Source: CAD feature listing. Evaluate the final solid. Frame: model axes, mm. A direction names the side the tool comes from. Coordinates: 2 decimals unless noted, no trailing zeros. Loops run counter-clockwise (first coordinate to the right, second up) from the corner with the lowest first, then second, coordinate; pieces in that order, holes last. Notation, with made-up numbers: M 57.5,86 L 68.5,86 A22 cw 68.5,123 Z; hole C 47.5,56 d11. An arc over 180 degrees is marked long. Write each question's results on one line, items separated by ' | '. Start each with the question number.
from build123d import *

# Parameters (mm, degrees)
F1_DEPTH  = 20
F2_R      = 3
F4_DEPTH  = 10.001
F5_DEPTH  = 6.5
F6_ANGLE  = -90
F7_R      = 2.25
F8_DEPTH  = 5.5
F9_R      = 3.75
F9_R_2    = 2.25
F10_DEPTH = 4


with BuildPart() as f1:
    # F0 (on Top) → F1 (new body)
    with BuildSketch(Plane.XY):
        Polygon((-15.7, 0), (0, 0), (15.7, 0), (15.7, 29.4), (10.2, 29.4), (9.7, 28), (10.2, 27.4), (10.2, 8), (3.1, 8), (2.1, 10), (0, 10), (-2.1, 10), (-3.1, 8), (-10.2, 8), (-10.2, 27.4), (-9.7, 28), (-10.2, 29.4), (-15.7, 29.4), align=None)
    extrude(amount=F1_DEPTH)

    # F2
    f2_edges = [f1.edges().sort_by_distance(p)[0] for p in [
        (12.95, 29.4, 20),
        (-12.95, 29.4, 20),
        (-12.95, 29.4, 0),
        (12.95, 29.4, 0),
    ]]
    fillet(f2_edges, radius=F2_R)

    # F3 (on face) → F4 (cut, through all)
    with BuildSketch(Plane(origin=(0, 10, 0), x_dir=(-1, 0, 0), z_dir=(0, 1, 0))):
        with BuildLine():
            ThreePointArc((5.95, 10), (4.5551315688, 12.0811655388), (2.1, 11.581929202))
            Line((2.1, 11.581929202), (2.1, 8.418070798))
            ThreePointArc((2.1, 8.418070798), (4.5551315688, 7.9188344612), (5.95, 10))
        make_face()
        with BuildLine():
            Line((2.1, 8.418070798), (2.1, 11.581929202))
            ThreePointArc((2.1, 11.581929202), (1.45, 10), (2.1, 8.418070798))
        make_face()
    extrude(amount=-F4_DEPTH, mode=Mode.SUBTRACT)

    # F3 (on face) → F5 (cut)
    with BuildSketch(Plane(origin=(0, 10, 0), x_dir=(-1, 0, 0), z_dir=(0, 1, 0))):
        with BuildLine():
            ThreePointArc((2.1, 6.6084664236), (5.7077973005, 6.8327851352), (7.45, 10))
            ThreePointArc((7.45, 10), (5.7077973005, 13.1672148648), (2.1, 13.3915335764))
            Line((2.1, 13.3915335764), (2.1, 11.581929202))
            ThreePointArc((2.1, 11.581929202), (4.5551315688, 12.0811655388), (5.95, 10))
            ThreePointArc((5.95, 10), (4.5551315688, 7.9188344612), (2.1, 8.418070798))
            Line((2.1, 8.418070798), (2.1, 6.6084664236))
        make_face()
        with BuildLine():
            Line((2.1, 11.581929202), (2.1, 13.3915335764))
            ThreePointArc((2.1, 13.3915335764), (-0.05, 10), (2.1, 6.6084664236))
            Line((2.1, 6.6084664236), (2.1, 8.418070798))
            ThreePointArc((2.1, 8.418070798), (1.45, 10), (2.1, 11.581929202))
        make_face()
    extrude(amount=-F5_DEPTH, mode=Mode.SUBTRACT)


with BuildPart() as f1_1:
    # F6: moved
    add(f1.part.rotate(Axis((0, 0, 0), (-1, 0, 0)), F6_ANGLE))

    # F7 (on face) → F8 (cut, through all)
    with BuildSketch(Plane.YZ.offset(-10.2)):
        with Locations((-10, 18)):
            Circle(F7_R)
    extrude(amount=-F8_DEPTH, mode=Mode.SUBTRACT)

    # F9 (on face) → F10 (cut)
    with BuildSketch(Plane(origin=(-15.7, 0, 0), x_dir=(0, -1, 0), z_dir=(-1, 0, 0))):
        with Locations((10, 18)):
            Circle(F9_R)
        with Locations((10, 18)):
            Circle(F9_R_2, mode=Mode.SUBTRACT)
    extrude(amount=-F10_DEPTH, mode=Mode.SUBTRACT)


solid = f1_1.part
Item 1: Line query: probe 1 along X at (y, z) = (-10, 2.5); probe 2 along X at (y, z) = (-14, 18.5); probe 3 along Z at (x, y) = (-11, -10). Output: solid intervals per line, ascending.
Item 2: Cut plane C-C (z = 5.5). Output: boundary loops of the cut face in (x, y), then the cut area to 3 significant figures.
Item 3: Access query for faces 1 (the cylindrical face through (-13.73, -9.19, 14.34)), 2 (the flat face through (-9.946, -9.866, 28.69)), 3 (the flat face through (-3.6, -7.6, 3.5)), 4 (the flat face through (-8, -10, 8)), 5 (the cylindrical face through (-12.74, -0.9, 28.54)). Directions: +Z, -Z, +X, -X, +Y, -Y. A direction counts if a zero-diameter tool reaches every point of the face in a straight line with its end or side. Return the directions, or none.
Item 4: Cut plane D-D (y = -4.75). Output: boundary loops of the cut face in (x, z).
Item 5: First-contact query: pin 1 Ø2 at (x, y) = (-4.5, -10.5) entering from +Z (3 decimals); pin 2 Ø3.5 at (x, y) = (6, -13.5) entering from +Z; pin 3 Ø1.3 at (x, y) = (1, -8.5) entering from +Z. Flat tips, straight axial feed; report the tip coordinate or a pass-through.
Item 6: Cut plane A-A (z = 12.75). Output: boundary loops of the cut face in (x, y), then the cut area to 3 significant figures.
Item 7: Cut plane B-B (x = -11). Output: boundary loops of the cut face in (y, z).
Item 8: Mould query, pull axis Y, two halves, no side actions, for faces 6 (the flat face through (0, -10, 0)), 7 (the flat face through (-11.7, -12, 16)), 8 (the cylindrical face through (12.66, -0.9, 28.54)). Classes: +Y half, -Y half, draft (parallel to the pull), parting line (faces both ways), or undercut.
Response values:
1) probe 1: x = -15.7 to -5.95, -1.45 to 15.7 | probe 2: x = -15.7 to -10.2, 10.2 to 15.7 | probe 3: z = 0 to 15.75, 20.25 to 29.4
2) outline: M -15.7,-20 L 15.7,-20 L 15.7,0 L -15.7,0 Z; hole C -3.7,-10 d7.5 | area: 584 mm2
3) face 1: -X | face 2: +Z, +Y, -Y | face 3: +Z | face 4: +Y, -Y | face 5: +Z, +X, -X, +Y
4) outline: M -15.7,0 L 15.7,0 L 15.7,29.4 L 10.2,29.4 L 9.7,28 L 10.2,27.4 L 10.2,8 L 3.1,8 L 2.1,10 L -2.1,10 L -3.1,8 L -10.2,8 L -10.2,27.4 L -9.7,28 L -10.2,29.4 L -15.7,29.4 Z
5) pin 1: passes through | pin 2: stops at z = 8 | pin 3: stops at z = 10
6) outline: M -15.7,-20 L -10.2,-20 L -10.2,0 L -15.7,0 Z; M 10.2,-20 L 15.7,-20 L 15.7,0 L 10.2,0 Z | area: 220 mm2
7) outline: M -20,0 L 0,0 L 0,26.4 A3 ccw -3,29.4 L -17,29.4 A3 ccw -20,26.4 Z; hole C -10,18 d4.5
8) face 6: draft | face 7: undercut | face 8: +Y half
